Input: part model. Units: mm. Frame: model coordinates. Face numbers are marked on the shaded views. Give positions to 0.01 mm unless a question says otherwise; leave off trailing zeros. Loops run counter-clockwise (first coordinate to the right, second up) from the corner with the lowest first, then second, coordinate; pieces in that order, holes last.
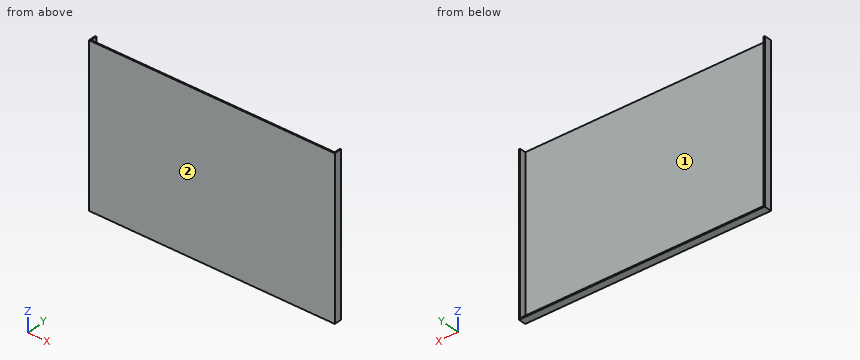
from build123d import *

# Parameters (mm, degrees)
SZKIC1_W                    = 387
SZKIC1_H                    = 1.85
DODANIE_WYCI_GNI_CIE1_DEPTH = 248
DODANIE_WYCI_GNI_CIE2_DEPTH = 10


with BuildPart() as part:
    # Szkic1 → Dodanie-wyciągnięcie1 (new body)
    with BuildSketch(Plane.XY):
        Rectangle(SZKIC1_W, SZKIC1_H)
    extrude(amount=DODANIE_WYCI_GNI_CIE1_DEPTH)

    # Szkic3 → Dodanie-wyciągnięcie2 (add)
    with BuildSketch(Plane(origin=(0, 0.925, 0), x_dir=(1, 0, 0), z_dir=(0, 1, 0))):
        Polygon((193.5, -248), (193.5, 0), (-193.5, 0), (-193.5, -248), (-191.65, -248), (-191.65, -1.85), (191.65, -1.85), (191.65, -248), align=None)
    extrude(amount=DODANIE_WYCI_GNI_CIE2_DEPTH)


solid = part.part
(1) Pin query (flat end, axial travel): pin 1 Ø1 at (x, y) = (-1.5, 5.5) entering from +Z. Return the tip coordinate at first contact, or that it passes through.
Values follow:
pin 1: stops at z = 1.85
(2) Cut plane C-C (x = -149.5). Return the cut outline in (y, z) (3 decimals).
Values follow:
outline: (-0.925, 0) - (10.925, 0) - (10.925, 1.85) - (0.925, 1.85) - (0.925, 248) - (-0.925, 248) - close
(3) Cut plane B-B (z = 113). Return the cut outline in (x, y) (3 decimals).
Values follow:
outline: (-193.5, -0.925) - (193.5, -0.925) - (193.5, 10.925) - (191.65, 10.925) - (191.65, 0.925) - (-191.65, 0.925) - (-191.65, 10.925) - (-193.5, 10.925) - close
(4) Cut plane A-A (y = 7.75). Return the cut outline in (x, z), and give its area (3 significant figures).
Values follow:
outline: (-193.5, 0) - (193.5, 0) - (193.5, 248) - (191.65, 248) - (191.65, 1.85) - (-191.65, 1.85) - (-191.65, 248) - (-193.5, 248) - close
area: 1,630 mm2
(5) Mould query, pull axis X, two halves, no side actions, for the marked faces 1 and 2. Classes: +X half, -X half, draft (parallel to the pull), parting line (faces both ways), or undercut.
Values follow:
face 1: undercut
face 2: draft
(6) Ray query, probe 1 along X at (y, z) = (8.5, 179.5); probe 2 along Y at (x, z) = (-87.5, 199) (3 decimals); probe 3 along Z at (x, y) = (50.5, 7). Return the intervals inside material, ascending.
Values follow:
probe 1: x = -193.5 to -191.65, 191.65 to 193.5
probe 2: y = -0.925 to 0.925
probe 3: z = 0 to 1.85
